```python
from build123d import *

# Parameters (mm, degrees)
F0_W     = 127
F0_H     = 76.2
F1_DEPTH = 12.7
F3_DEPTH = 25.4
F4_R     = 12.7
F5_DEPTH = 12.701


with BuildPart() as f1:
    # F0 (on Top) → F1 (new body)
    with BuildSketch(Plane.XY):
        Rectangle(F0_W, F0_H)
    extrude(amount=F1_DEPTH)

    # F2 (on face) → F3 (join)
    with BuildSketch(Plane.XY.offset(12.7)):
        with BuildLine():
            Line((31.75, 7.62), (31.75, 38.1))
            ThreePointArc((31.75, 38.1), (0, 6.35), (-31.75, 38.1))
            Line((-31.75, 38.1), (-31.75, 7.62))
            ThreePointArc((-31.75, 7.62), (-35.4697438789, -1.3602561211), (-44.45, -5.08))
            Line((-44.45, -5.08), (-50.8, -5.08))
            Line((-50.8, -5.08), (-50.8, -38.1))
            Line((-50.8, -38.1), (-38.7925468385, -38.1))
            Line((-38.7925468385, -38.1), (-38.7925468385, -25.4))
            Line((-38.7925468385, -25.4), (37.4074531615, -25.4))
            Line((37.4074531615, -25.4), (37.4074531615, -38.1))
            Line((37.4074531615, -38.1), (50.8, -38.1))
            Line((50.8, -38.1), (50.8, -5.08))
            Line((50.8, -5.08), (44.45, -5.08))
            ThreePointArc((44.45, -5.08), (35.4697438789, -1.3602561211), (31.75, 7.62))
        make_face()
    extrude(amount=F3_DEPTH)

    # F4
    f4_edges = [f1.edges().sort_by_distance(p)[0] for p in [
        (-63.5, 38.1, 6.35),
        (63.5, 38.1, 6.35),
    ]]
    fillet(f4_edges, radius=F4_R)

    # F5 (cut, through all): a face of the model
    f5_faces = [f1.faces().sort_by_distance(p)[0] for p in [
        (0, 24.6248814849, 12.7),
    ]]
    extrude(f5_faces, amount=-F5_DEPTH, mode=Mode.SUBTRACT)


solid = f1.part
```
The model under review builds one solid part; all positions refer to its coordinate system, in mm. A direction names the side the tool comes from. Round coordinates to 2 decimals unless told otherwise and drop trailing zeros. Loops run counter-clockwise (first coordinate to the right, second up) from the corner with the lowest first, then second, coordinate; pieces in that order, holes last.
Item 1: For faces 4 (the face through (-50.8, -21, 25)), 5 (the face through (-48, -5.08, 25)), 6 (the face through (-1, -32, 12.7)), 7 (the face through (48, -5.08, 25)), list the 3-axis set-ups (+Z, -Z, +X, -X, +Y, -Y) from which the entire face can be reached by the end or side of a thin tool; tool diameter is ignored.
Determined:
face 4: +Z, -X, +Y, -Y
face 5: +Z, -X, +Y
face 6: +Z, -Y
face 7: +Z, +X, +Y
Item 2: Take a section at C-C (y = -8.5). Write out the cut boundary in (x, z), then the cut area to 3 significant figures.
Determined:
outline: (-63.5, 0) - (63.5, 0) - (63.5, 12.7) - (50.8, 12.7) - (50.8, 38.1) - (-50.8, 38.1) - (-50.8, 12.7) - (-63.5, 12.7) - close
area: 4,190 mm2
Item 3: Take a section at A-A (z = 3.5). Write out the cut boundary in (x, y).
Determined:
outline: (-63.5, -38.1) - (63.5, -38.1) - (63.5, 25.4) arc R12.7 ccw to (50.8, 38.1) - (31.75, 38.1) arc R31.75 cw to (-31.75, 38.1) - (-50.8, 38.1) arc R12.7 ccw to (-63.5, 25.4) - close
Item 4: Mouldability with a two-part tool opening along X and no side actions: class faces 1 (the face through (41, 38.1, 6)), 2 (the face through (-1, -25.4, 25)), 3 (the face through (31.75, 23, 25)) as released by +X, released by -X, zero draft, split by the parting line, or undercut.
Determined:
face 1: zero draft
face 2: undercut
face 3: released by +X
Item 5: Clearance check with flat-ended pins moving along their axes: pin 1 Ø4 at (x, y) = (-28, 27) entering from +Z; pin 2 Ø20.5 at (y, z) = (17, 31.5) entering from -X; pin 3 Ø5 at (y, z) = (-26.5, 19.5) entering from -X; pin 4 Ø3 at (x, z) = (-46.5, 30) entering from +Y. State where each tip first meets the part, or that it passes through.
Determined:
pin 1: stops at z = 38.1
pin 2: stops at x = -31.78
pin 3: stops at x = -50.8
pin 4: stops at y = -5.08
Item 6: Take a section at D-D (z = 17). Write out the cut boundary in (x, y), then the cut area to 3 significant figures.
Determined:
outline: (-50.8, -38.1) - (-38.79, -38.1) - (-38.79, -25.4) - (37.41, -25.4) - (37.41, -38.1) - (50.8, -38.1) - (50.8, -5.08) - (44.45, -5.08) arc R12.7 cw to (31.75, 7.62) - (31.75, 38.1) arc R31.75 cw to (-31.75, 38.1) - (-31.75, 7.62) arc R12.7 cw to (-44.45, -5.08) - (-50.8, -5.08) - close
area: 3,610 mm2
Item 7: Take a section at B-B (x = 0). Write out the cut boundary in (y, z), then the cut area to 3 significant figures.
Determined:
outline: (-38.1, 0) - (6.35, 0) - (6.35, 38.1) - (-25.4, 38.1) - (-25.4, 12.7) - (-38.1, 12.7) - close
area: 1,370 mm2
Item 8: For line 1 (X direction, y = -35, z = 16); line 2 (Z direction, x = -54.5, y = -15); line 3 (Y direction, x = 49, z = 23.5), list the stretches that pass through material, from the lowest coordinate up.
Determined:
line 1: x = -50.8 to -38.79, 37.41 to 50.8
line 2: z = 0 to 12.7
line 3: y = -38.1 to -5.08
